```python
from build123d import *
from OCP.BRepFilletAPI import BRepFilletAPI_MakeChamfer

# Parameters (mm, degrees)
SKETCH1_R           = 2.05
BOSS_EXTRUDE1_DEPTH = 10
CHAMFER1_SIZE       = 0.4
CHAMFER1_SIZE2      = 0.476701437


with BuildPart() as part:
    # Sketch1 → Boss-Extrude1 (new body)
    with BuildSketch(Plane(origin=(0, 0, 0), x_dir=(1, 0, 0), z_dir=(0, 1, 0))):
        with BuildLine():
            Line((-4.05, -3.955), (-4.05, 3.955))
            ThreePointArc((-4.05, 3.955), (0, 8.005), (4.05, 3.955))
            Line((4.05, 3.955), (4.05, -3.955))
            ThreePointArc((4.05, -3.955), (0, -8.005), (-4.05, -3.955))
        make_face()
        with Locations(Location((0, 3.955, 0), (0, 0, 270))):
            Circle(SKETCH1_R, mode=Mode.SUBTRACT)
        with Locations(Location((0, -3.955, 0), (0, 0, 270))):
            Circle(SKETCH1_R, mode=Mode.SUBTRACT)
    extrude(amount=BOSS_EXTRUDE1_DEPTH)

    # Chamfer1: one chamfer whose edges measure the first distance from different faces: ONE call of the kernel's chamfer builder (chamfer() names one face for all edges)
    chamfer1_edges_1 = [part.edges().sort_by_distance(p)[0] for p in [
        (0, 0, -6.005),
    ]]
    chamfer1_side_1 = [part.faces().sort_by_distance(p)[0] for p in [
        (0, 5, -6.005),
    ]]
    chamfer1_edges_2 = [part.edges().sort_by_distance(p)[0] for p in [
        (0, 10, -6.005),
        (0, 10, 1.905),
    ]]
    chamfer1_side_2 = [part.faces().sort_by_distance(p)[0] for p in [
        (0, 10, 0),
    ]]
    chamfer1_edges_3 = [part.edges().sort_by_distance(p)[0] for p in [
        (0, 10, -8.005),
    ]]
    chamfer1_side_3 = [part.faces().sort_by_distance(p)[0] for p in [
        (0, 5, -8.005),
    ]]
    chamfer1_edges_4 = [part.edges().sort_by_distance(p)[0] for p in [
        (0, 0, 1.905),
    ]]
    chamfer1_side_4 = [part.faces().sort_by_distance(p)[0] for p in [
        (0, 5, 1.905),
    ]]
    chamfer1_edges_5 = [part.edges().sort_by_distance(p)[0] for p in [
        (-4.05, 10, 0),
    ]]
    chamfer1_side_5 = [part.faces().sort_by_distance(p)[0] for p in [
        (-4.05, 5, 0),
    ]]
    chamfer1_edges_6 = [part.edges().sort_by_distance(p)[0] for p in [
        (0, 10, 8.005),
    ]]
    chamfer1_side_6 = [part.faces().sort_by_distance(p)[0] for p in [
        (0, 5, 8.005),
    ]]
    chamfer1_edges_7 = [part.edges().sort_by_distance(p)[0] for p in [
        (4.05, 10, 0),
    ]]
    chamfer1_side_7 = [part.faces().sort_by_distance(p)[0] for p in [
        (4.05, 5, 0),
    ]]
    chamfer1 = BRepFilletAPI_MakeChamfer(part.part.solid().wrapped)
    for e in chamfer1_edges_1:
        chamfer1.Add(CHAMFER1_SIZE, CHAMFER1_SIZE2, e.wrapped, chamfer1_side_1[0].wrapped)  # the first distance lies on this face
    for e in chamfer1_edges_2:
        chamfer1.Add(CHAMFER1_SIZE, CHAMFER1_SIZE2, e.wrapped, chamfer1_side_2[0].wrapped)  # the first distance lies on this face
    for e in chamfer1_edges_3:
        chamfer1.Add(CHAMFER1_SIZE, CHAMFER1_SIZE2, e.wrapped, chamfer1_side_3[0].wrapped)  # the first distance lies on this face
    for e in chamfer1_edges_4:
        chamfer1.Add(CHAMFER1_SIZE, CHAMFER1_SIZE2, e.wrapped, chamfer1_side_4[0].wrapped)  # the first distance lies on this face
    for e in chamfer1_edges_5:
        chamfer1.Add(CHAMFER1_SIZE, CHAMFER1_SIZE2, e.wrapped, chamfer1_side_5[0].wrapped)  # the first distance lies on this face
    for e in chamfer1_edges_6:
        chamfer1.Add(CHAMFER1_SIZE, CHAMFER1_SIZE2, e.wrapped, chamfer1_side_6[0].wrapped)  # the first distance lies on this face
    for e in chamfer1_edges_7:
        chamfer1.Add(CHAMFER1_SIZE, CHAMFER1_SIZE2, e.wrapped, chamfer1_side_7[0].wrapped)  # the first distance lies on this face
    add(Compound.cast(chamfer1.Shape()), mode=Mode.REPLACE)


solid = part.part
```
Work out the finished part from the listing and answer in its coordinate system (mm). Give positions to 0.01 mm unless a question says otherwise; leave off trailing zeros. Order: outer loops, then holes, each group sorted by start corner. A loop starts at its lowest first (then second) coordinate and runs counter-clockwise, first axis right, second up. Notation, with made-up numbers: (19, 57.5) -> (43, 57.5) arc R26 cw to (43, 79.5) -> close; hole circle Ø2 at (81.5, 58). An arc over 180 degrees is marked (long way). Answer as CSV lines item,"result". Start each with the question number.
(1) Section A-A, the plane x = 0 is taken. Write down the section's boundary in (y, z) (3 decimals).
(2) Section B-B, the plane y = 6.5 is taken. Write down the section's boundary in (x, z) (3 decimals).
(3) Consider line 1 along Z through (x, y) = (1, 9.5); line 2 along Z through (x, y) = (-0.5, 4.25); line 3 along X through (y, z) = (0.5, -4). Determine where each line is inside the solid, lowest interval first.
(4) For a pull along Z with two mould halves and no side action, classify faces 1 (the flat face through (-4.05, 5, 0)), 2 (the cylindrical face through (0.09, 4.898, -6.003)), 3 (the cylindrical face through (0.089, 4.733, 8.004)), 4 (the cylindrical face through (-0.089, 4.733, -8.004)) as released by +Z, released by -Z, zero draft, split by the parting line, or undercut.
(5) This flat-tipped pin is pushed along its axis until it touches: pin 1 Ø4 at (x, z) = (-1.5, 2.5) entering from -Y. Where does it stop, or does it pass through?
Entries:
1,outline,"(0, -8.005) -> (9.6, -8.005) -> (10, -7.528) -> (10, -6.405) -> (9.523, -6.005) -> (0.4, -6.005) -> (0, -6.482) -> close; (0, -1.428) -> (0.4, -1.905) -> (9.523, -1.905) -> (10, -1.505) -> (10, 1.505) -> (9.523, 1.905) -> (0.4, 1.905) -> (0, 1.428) -> close; (0, 6.482) -> (0.4, 6.005) -> (9.523, 6.005) -> (10, 6.405) -> (10, 7.528) -> (9.6, 8.005) -> (0, 8.005) -> close"
2,outline,"(-4.05, -3.955) arc R4.05 ccw to (4.05, -3.955) -> (4.05, 3.955) arc R4.05 ccw to (-4.05, 3.955) -> close; hole circle Ø4.1 at (0, -3.955); hole circle Ø4.1 at (0, 3.955)"
3,line 1,"-7.88 to -5.74, -2.17 to 2.17, 5.74 to 7.88"
3,line 2,"-7.97 to -5.94, -1.97 to 1.97, 5.94 to 7.97"
3,line 3,"-4.05 to -2.05, 2.05 to 4.05"
4,face 1,"zero draft"
4,face 2,"undercut"
4,face 3,"released by +Z"
4,face 4,"released by -Z"
5,pin 1,"y = 0"
